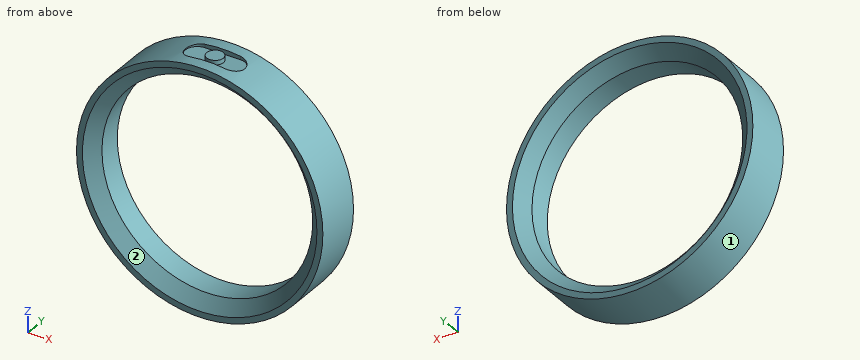
```python
from build123d import *

# Parameters (mm, degrees)
F0_R          = 10.375
F0_R_2        = 8.875
F1_DEPTH      = 2
F1_DEPTH_BACK = 2
F2_SIZE       = 1
F4_START      = 9.975
F3_R          = 0.7
F4_DEPTH      = 15.025


with BuildPart() as f1:
    # F0 (on Front) → F1 (new body, two sides)
    with BuildSketch(Plane.XZ) as f1_sk:
        Circle(F0_R)
        Circle(F0_R_2, mode=Mode.SUBTRACT)
    extrude(amount=F1_DEPTH)
    extrude(f1_sk.sketch, amount=-F1_DEPTH_BACK)

    # F2
    f2_edges = [f1.edges().sort_by_distance(p)[0] for p in [
        (-8.875, -2, 0),
        (-8.875, 2, 0),
    ]]
    chamfer(f2_edges, length=F2_SIZE)

    # F3 (on Top) → F4 (cut)
    with BuildSketch(Plane.XY.offset(F4_START)):
        with BuildLine():
            Line((-1.5, -1), (1.5, -1))
            ThreePointArc((1.5, -1), (2.2071067812, -0.7071067812), (2.5, 0))
            ThreePointArc((2.5, 0), (2.2071067812, 0.7071067812), (1.5, 1))
            Line((1.5, 1), (-1.5, 1))
            ThreePointArc((-1.5, 1), (-2.2071067812, 0.7071067812), (-2.5, 0))
            ThreePointArc((-2.5, 0), (-2.2071067812, -0.7071067812), (-1.5, -1))
        make_face()
        Circle(F3_R, mode=Mode.SUBTRACT)
    extrude(amount=F4_DEPTH, mode=Mode.SUBTRACT)


solid = f1.part
```
Geometry: final body of the model. Coordinates: model frame, mm. Face numbers are marked on the shaded views. Round coordinates to 2 decimals unless told otherwise and drop trailing zeros. Loops run counter-clockwise (first coordinate to the right, second up) from the corner with the lowest first, then second, coordinate; pieces in that order, holes last. Notation, with made-up numbers: (55, -22) -> (85, -22) arc R11 cw to (85, -15) -> close; hole circle Ø10 at (-37.75, 18.25). An arc over 180 degrees is marked (long way). Use one line per item in the form item = value. Start each with the question number.
1) Line query: L1, parallel to Z at x = 0, y = 0.05 (3 decimals); L2, parallel to X at y = -0.6, z = -4.5; L3, parallel to Z at x = -7.75, y = -0.55. Output: solid intervals per line, ascending.
2) Draft query along Z for the marked faces 1 and 2. Return one class per face: released by +Z, released by -Z, zero draft, split by the parting line, or undercut.
3) First-contact query: P1, Ø1, axis at x = 3, y = 0, coming from the +Z side; P2, Ø8, axis at x = -0.5, z = -5, coming from the +Y side; P3, Ø1, axis at x = -1, y = 1, coming from the -Z side. Flat tips, straight axial feed; report the tip coordinate or a pass-through.
4) Section C-C on y = -1.4. Output: boundary loops of the cut face in (x, z) (3 decimals), then the cut area to 3 significant figures.
5) Section A-A on x = 0. Output: boundary loops of the cut face in (y, z) (3 decimals), then the cut area to 3 significant figures.
6) Section B-B on z = 0. Output: boundary loops of the cut face in (x, y) (3 decimals).
Response:
q1.L1 = -10.375 to -8.875, 8.875 to 10.375
q1.L2 = -9.35 to -7.65, 7.65 to 9.35
q1.L3 = -6.9 to -4.32, 4.32 to 6.9
q2.face_1 = split by the parting line
q2.face_2 = undercut
q3.P1 = 10.07
q3.P2 = 1.15
q3.P3 = -10.36
q4.outline = circle Ø20.75 at (0, 0); hole circle Ø18.55 at (0, 0)
q4.area = 67.9 mm^2
q5.outline = (-2, -10.375) -> (2, -10.375) -> (2, -9.875) -> (1, -8.875) -> (-1, -8.875) -> (-2, -9.875) -> close; (-2, 9.875) -> (-1, 8.875) -> (1, 8.875) -> (2, 9.875) -> (2, 10.375) -> (1, 10.375) -> (1, 9.975) -> (0.7, 9.975) -> (0.7, 10.375) -> (-0.7, 10.375) -> (-0.7, 9.975) -> (-1, 9.975) -> (-1, 10.375) -> (-2, 10.375) -> close
q5.area = 9.76 mm^2
q6.outline = (-10.375, -2) -> (-9.875, -2) -> (-8.875, -1) -> (-8.875, 1) -> (-9.875, 2) -> (-10.375, 2) -> close; (8.875, -1) -> (9.875, -2) -> (10.375, -2) -> (10.375, 2) -> (9.875, 2) -> (8.875, 1) -> close
